Can you work these out from the model? Positions are in its coordinate system, mm. Face numbers are marked on the shaded views. Round coordinates to 2 decimals unless told otherwise and drop trailing zeros. Loops run counter-clockwise (first coordinate to the right, second up) from the corner with the lowest first, then second, coordinate; pieces in that order, holes last. Notation, with made-up numbers: M 38.5,22.25 L 60.5,22.25 A22 cw 60.5,59.25 Z; hole C -18.75,-26 d6. An arc over 180 degrees is marked long. Answer as CSV lines item,"result".
from build123d import *

# Parameters (mm, degrees)
BOSS_EXTRUDE1_DEPTH = 6.35
CUT_EXTRUDE1_DEPTH  = 58.404294318


with BuildPart() as part:
    # Sketch13 → Boss-Extrude1 (new body)
    with BuildSketch(Plane.XY):
        with BuildLine():
            Line((11.551437691, 43.580058654), (2.682196049, 13.0624672))
            ThreePointArc((2.682196049, 13.0624672), (-4.12074162, 12.682338645), (-9.847867764, 8.991202672))
            Line((-9.847867764, 8.991202672), (-34.961025172, 28.467243349))
            ThreePointArc((-34.961025172, 28.467243349), (-13.932031191, 42.878383037), (11.551437691, 43.580058654))
        make_face()
    extrude(amount=-BOSS_EXTRUDE1_DEPTH)

    # Sketch15 → Cut-Extrude1 (cut, through all)
    with BuildSketch(Plane.XY):
        with BuildLine():
            Line((7.682261651, 30.266864763), (4.669640038, 19.900932781))
            ThreePointArc((4.669640038, 19.900932781), (2.491973647, 26.154562688), (7.682261651, 30.266864763))
        make_face()
        with BuildLine():
            Line((-24.005496972, 19.970887857), (-15.475292944, 13.355447276))
            ThreePointArc((-15.475292944, 13.355447276), (-17.389315258, 19.694740336), (-24.005496972, 19.970887857))
        make_face()
    extrude(amount=-CUT_EXTRUDE1_DEPTH, mode=Mode.SUBTRACT)


solid = part.part
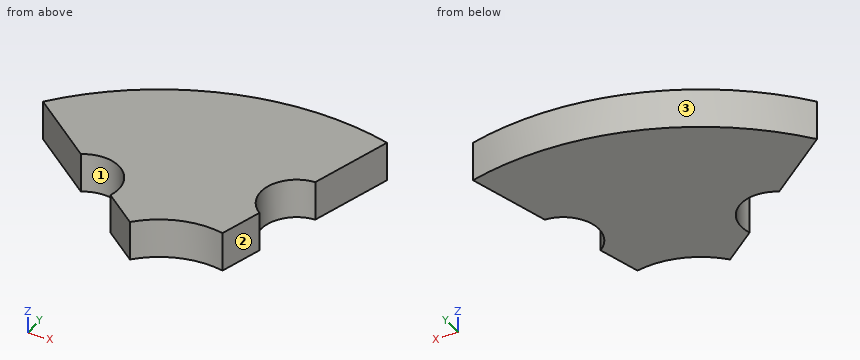
Item 1: If I drill on line 1 along X through (y, z) = (15.5, -1); line 2 along X through (y, z) = (12, -2); line 3 along Y through (x, z) = (-7, -0.75), over which ranges is the centre line in solid material (lowest first)? Write a range as from..to.
Output:
line 1,"x = -15.19..3.39"
line 2,"x = -13.73..-5.82"
line 3,"y = 11.35..44.54"
Item 2: We'd pull the mould along Y, two halves only. Please class the marked faces 1, 2 and 3: released by +Y, released by -Y, zero draft, split by the parting line, or undercut.
Output:
face 1,"undercut"
face 2,"released by -Y"
face 3,"released by +Y"
Item 3: Will these pins go through, and if not, where does the flat tip stop? pin 1 (1 mm diameter, centred on y = 24, z = -1, fed in from -X); pin 2 (3 mm diameter, centred on y = 39.5, z = -2.5, fed in from -X); pin 3 (1 mm diameter, centred on y = 26.5, z = -1.5, fed in from +X).
Output:
pin 1,"stops at x = -29.85"
pin 2,"stops at x = -24.26"
pin 3,"stops at x = 2.81"
Item 4: If we section it at A-A on z = -3.25: Write out the boundary of the cut face in (x, y) (1 decimal), then the cut area to 3 significant figures.
Output:
outline,"M -35,28.5 L -24,20 A5.7 cw -15.5,13.4 L -9.8,9 A13.3 cw 2.7,13.1 L 4.7,19.9 A5.7 cw 7.7,30.3 L 11.6,43.6 A45.1 ccw Z"
area,"979 mm2"
Item 5: If we section it at B-B on x = -31: Write out the boundary of the cut face in (y, z), then the cut area to 3 significant figures.
Output:
outline,"M 25.4,-6.35 L 32.74,-6.35 L 32.74,0 L 25.4,0 Z"
area,"46.6 mm2"
Item 6: If we section it at C-C on y = 14.5: Write out the boundary of the cut face in (x, z).
Output:
outline,"M -15.22,-6.35 L 3.1,-6.35 L 3.1,0 L -15.22,0 Z"
